Design review of the part built by this model. Coordinates are the model's own, in mm. A direction names the side the tool comes from. Coordinates: 2 decimals unless noted, no trailing zeros.
Q1. Take a section at A-A, the plane y = -1.25. State how many separate pieces and enclosed holes the cut face has, plus the area to 3 significant figures.
Q2. For pin 1 Ø4 at (x, z) = (116.205, 12.7) entering from +Y, flat-tipped, find the tip position at first contact; note if it passes through.
Q3. The part is to be moulded in two halves that separate along Z. For faces 1 (the cylindrical face through (152.494, 0.044, -23.49)), 2 (the flat face through (13, 0, 25.4)), 3 (the cylindrical face through (73.76, 0.04, 9.01)), say which applies: released by +Z, released by -Z, zero draft, split by the parting line, or undercut.
Q4. For L1, parallel to X at y = -0.25, z = 14.5 (3 decimals); L2, parallel to Z at x = -71.5, y = -1.75; L3, parallel to Z at x = -23, y = 0.5, list the stretches that pass through material, from the lowest coordinate up.
Q5. For faces 4 (the flat face through (-26.09, 0.04, 6.05)), 5 (the flat face through (137.681, 0.044, 9.184)), list the 3-axis set-ups (+Z, -Z, +X, -X, +Y, -Y) from which the entire face can be reached by the end or side of a thin tool; tool diameter is ignored.
from build123d import *

# Parameters (mm, degrees)
SKETCH1_R           = 3.175
BOSS_EXTRUDE1_DEPTH = 3.175
FILLET1_R           = 2.54
FILLET2_R           = 6.35


with BuildPart() as part:
    # Sketch1 → Boss-Extrude1 (new body, symmetric)
    with BuildSketch(Plane(origin=(0, 0, 0), x_dir=(1, 0, 0), z_dir=(0, 1, 0))):
        Polygon((121.465512242, -25.4), (154.305, 7.439487758), (154.305, 25.4), (-92.075, 25.4), (-92.075, -25.4), align=None)
        Polygon((-38.817248104, -20.32), (-73.366085229, -20.32), (-56.091666667, 14.592509095), align=None, mode=Mode.SUBTRACT)
        Polygon((-15.875, 14.592509095), (-15.875, -20.32), (-33.149418563, -20.32), align=None, mode=Mode.SUBTRACT)
        Polygon((22.200034711, -20.32), (0, -20.32), (0, 15.498543399), align=None, mode=Mode.SUBTRACT)
        with Locations((116.205, -12.7)):
            Circle(SKETCH1_R, mode=Mode.SUBTRACT)
        Polygon((72.576701378, -20.32), (28.176631956, -20.32), (50.376666667, 15.498543399), align=None, mode=Mode.SUBTRACT)
        Polygon((53.364965289, 20.32), (75.565, 20.32), (75.565, -15.498543399), align=None, mode=Mode.SUBTRACT)
        Polygon((-76.2, -14.592509095), (-76.2, 20.32), (-58.925581437, 20.32), align=None, mode=Mode.SUBTRACT)
        Polygon((-53.257751896, 20.32), (-18.708914771, 20.32), (-35.983333333, -14.592509095), align=None, mode=Mode.SUBTRACT)
        Polygon((2.988298622, 20.32), (47.388368044, 20.32), (25.188333333, -15.498543399), align=None, mode=Mode.SUBTRACT)
        with Locations((141.605, 12.7)):
            Circle(SKETCH1_R, mode=Mode.SUBTRACT)
    extrude(amount=BOSS_EXTRUDE1_DEPTH, both=True)

    # Fillet1
    fillet1_edges = [part.edges().sort_by_distance(p)[0] for p in [
        (-76.2, 0, -20.32),
        (-76.2, 0, 14.592509095),
        (-58.925581437, 0, -20.32),
        (2.988298622, 0, -20.32),
        (25.188333333, 0, 15.498543399),
        (47.388368044, 0, -20.32),
        (0, 0, -15.498543399),
        (0, 0, 20.32),
        (22.200034711, 0, 20.32),
        (72.576701378, 0, 20.32),
        (50.376666667, 0, -15.498543399),
        (28.176631956, 0, 20.32),
        (75.565, 0, 15.498543399),
        (75.565, 0, -20.32),
        (53.364965289, 0, -20.32),
        (-15.875, 0, 20.32),
        (-15.875, 0, -14.592509095),
        (-33.149418563, 0, 20.32),
        (-35.983333333, 0, 14.592509095),
        (-18.708914771, 0, -20.32),
        (-53.257751896, 0, -20.32),
        (-92.075, 0, 25.4),
        (-92.075, 0, -25.4),
        (-38.817248104, 0, 20.32),
        (-56.091666667, 0, -14.592509095),
        (-73.366085229, 0, 20.32),
    ]]
    fillet(fillet1_edges, radius=FILLET1_R)

    # Fillet2
    fillet2_edges = [part.edges().sort_by_distance(p)[0] for p in [
        (154.305, 0, -25.4),
        (154.305, 0, -7.439487758),
        (121.465512242, 0, 25.4),
    ]]
    fillet(fillet2_edges, radius=FILLET2_R)


solid = part.part
Responses:
1. separate pieces: 1
1. enclosed holes: 10
1. area: 7,850 mm2
2. pin 1: passes through
3. face 1: released by -Z
3. face 2: released by +Z
3. face 3: undercut
4. L1: x = -92.075 to -70.486, -41.697 to -30.27, -15.875 to 0, 18.593 to 31.784, 68.97 to 113.59, 118.82 to 132.366
4. L2: z = -25.4 to -20.32, 5.07 to 16.55, 19.01 to 25.4
4. L3: z = -25.4 to -20.32, -11.65 to -0.19, 20.32 to 25.4
5. face 4: +Y, -Y
5. face 5: +Z, +X, +Y, -Y
